```python
from build123d import *

# Parameters (mm, degrees)
SKETCH1_W           = 250
SKETCH1_H           = 100
BOSS_EXTRUDE1_DEPTH = 3
SKETCH2_R           = 1.8
CUT_EXTRUDE1_DEPTH  = 4
SKETCH3_W           = 25
SKETCH3_H           = 27
CUT_EXTRUDE2_DEPTH  = 4


with BuildPart() as part:
    # Sketch1 → Boss-Extrude1 (new body)
    with BuildSketch(Plane.XY):
        with Locations((125, 50)):
            Rectangle(SKETCH1_W, SKETCH1_H)
    extrude(amount=BOSS_EXTRUDE1_DEPTH)

    # Sketch2 → Cut-Extrude1 (cut, through all)
    with BuildSketch(Plane.XY.offset(3)):
        with Locations((6, 93)):
            Circle(SKETCH2_R)
        with Locations((80, 90)):
            Circle(SKETCH2_R)
        with Locations((240, 90)):
            Circle(SKETCH2_R)
        with Locations((240, 10)):
            Circle(SKETCH2_R)
        with Locations((80, 10)):
            Circle(SKETCH2_R)
        with Locations((6, 7)):
            Circle(SKETCH2_R)
    extrude(amount=-CUT_EXTRUDE1_DEPTH, mode=Mode.SUBTRACT)

    # Sketch3 → Cut-Extrude2 (cut, through all)
    with BuildSketch(Plane.XY.offset(3)):
        with Locations((85.5, 50)):
            Rectangle(SKETCH3_W, SKETCH3_H)
        with Locations((174.5, 50)):
            Rectangle(SKETCH3_W, SKETCH3_H)
    extrude(amount=-CUT_EXTRUDE2_DEPTH, mode=Mode.SUBTRACT)


solid = part.part
```
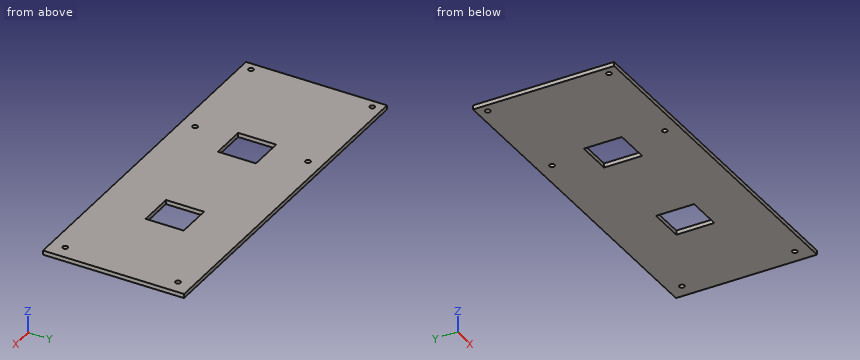
For this review, take the finished solid that the model builds, in its own axes (mm). Round coordinates to 2 decimals unless told otherwise and drop trailing zeros. Write each loop counter-clockwise with the first axis right and the second up, starting at its lowest first coordinate (ties: lowest second). Pieces come first, ordered by that corner, then holes.
1) Take a section at A-A on y = 47.5. Give the boundary of the cut face in (x, z).
Answer below:
outline: (0, 0) - (73, 0) - (73, 3) - (0, 3) - close; (98, 0) - (162, 0) - (162, 3) - (98, 3) - close; (187, 0) - (250, 0) - (250, 3) - (187, 3) - close
2) Take a section at B-B on z = 0.7. State how many separate pieces and enclosed holes the cut face has, then the cut area to 3 significant figures.
Answer below:
separate pieces: 1
enclosed holes: 8
area: 23,600 mm2
3) Insertion check: pin 1 Ø4.5 at (x, y) = (240, 90) entering from +Z; pin 2 Ø2 at (x, y) = (80, 10) entering from +Z. Each pin has a flat end and moves straight along its axis. Give the tip position at first contact, or say it passes through.
Answer below:
pin 1: stops at z = 3
pin 2: passes through
4) For line 1 along X through (y, z) = (90, 1.55); line 2 along X through (y, z) = (47, 1.05); line 3 along Y through (x, z) = (240, 1.6), list the stretches that pass through material, from the lowest coordinate up.
Answer below:
line 1: x = 0 to 78.2, 81.8 to 238.2, 241.8 to 250
line 2: x = 0 to 73, 98 to 162, 187 to 250
line 3: y = 0 to 8.2, 11.8 to 88.2, 91.8 to 100
5) Take a section at C-C on x = 169.5. Give the boundary of the cut face in (y, z).
Answer below:
outline: (0, 0) - (36.5, 0) - (36.5, 3) - (0, 3) - close; (63.5, 0) - (100, 0) - (100, 3) - (63.5, 3) - close
